Verification items for the finished model (mm, model axes). Give positions to 0.01 mm unless a question says otherwise; leave off trailing zeros. Order: outer loops, then holes, each group sorted by start corner. A loop starts at its lowest first (then second) coordinate and runs counter-clockwise, first axis right, second up.
(1) Sectioned sample at A-A on x = 34. Record the cut outline in (y, z).
(2) Scan lines: L1, parallel to Z at x = -24.5, y = 37; L2, parallel to Y at x = -35, z = -14; L3, parallel to Z at x = 4, y = 20.5. Record each from-to range of solid material in increasing order.
(3) Sectioned sample at B-B on z = -11.5. Record the cut outline in (x, y), plus the area to 3 significant figures.
(4) Gauge pin test, flat ends, axial feed: pin 1 (4 mm diameter, centred on x = 13, z = 21.5, fed in from -Y); pin 2 (12 mm diameter, centred on x = -10.5, z = -14.5, fed in from +Y); pin 3 (8 mm diameter, centred on x = -26, z = -19.5, fed in from +Y); pin 4 (8 mm diameter, centred on x = 28, y = 47.5, fed in from +Z). Record the tip position at first contact, or that the pin passes through.
(5) Sectioned sample at C-C on y = 66. Record the cut outline in (x, z).
```python
from build123d import *

# Parameters (mm, degrees)
F0_W     = 101.522006
F0_H     = 83.972574
F1_DEPTH = 102.4
F2_R     = 83.290368


with BuildPart() as f1:
    # F0 (on Front) → F1 (new body)
    with BuildSketch(Plane.XZ):
        Rectangle(F0_W, F0_H)
    extrude(amount=-F1_DEPTH)

    # F2
    f2_edges = [f1.edges().sort_by_distance(p)[0] for p in [
        (0, 102.4, 41.986287),
    ]]
    fillet(f2_edges, radius=F2_R)


solid = f1.part
```
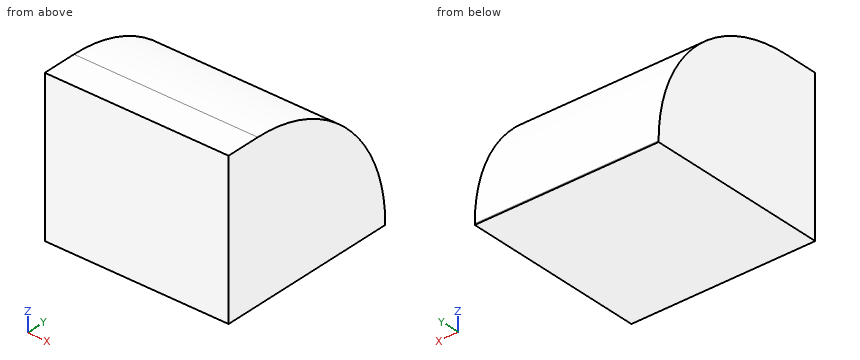
Ans:
1. outline: (0, -41.99) - (102.4, -41.99) - (102.4, -41.3) arc R83.29 ccw to (19.11, 41.99) - (0, 41.99) - close
2. L1: z = -41.99 to 40.04
2. L2: y = 0 to 97.8
2. L3: z = -41.99 to 41.97
3. outline: (-50.76, 0) - (50.76, 0) - (50.76, 96.88) - (-50.76, 96.88) - close
3. area: 9,840 mm2
4. pin 1: stops at y = 0
4. pin 2: stops at y = 99.76
4. pin 3: stops at y = 100.47
4. pin 4: stops at z = 38.34
5. outline: (-50.76, -41.99) - (50.76, -41.99) - (50.76, 27.53) - (-50.76, 27.53) - close
